from build123d import *

# Parameters (mm, degrees)
SKETCH1_R           = 1
BOSS_EXTRUDE1_DEPTH = 1
SKETCH2_R           = 1
BOSS_EXTRUDE2_DEPTH = 1
SKETCH3_R           = 1
BOSS_EXTRUDE3_DEPTH = 1


with BuildPart() as part:
    # Sketch1 → Boss-Extrude1 (new body)
    with BuildSketch(Plane(origin=(0, 0, 0), x_dir=(1, 0, 0), z_dir=(0, 1, 0))):
        with BuildLine():
            Line((-26.5, 3), (26.5, 3))
            ThreePointArc((26.5, 3), (29.222667474, 1.259794359), (28.786667416, -1.941945449))
            Line((28.786667416, -1.941945449), (2.247877744, -8.598102408))
            ThreePointArc((2.247877744, -8.598102408), (-0.45558898, -8.991146774), (-3.153897824, -8.56412735))
            Line((-3.153897824, -8.56412735), (-26.5, -3))
            ThreePointArc((-26.5, -3), (-29.5, 0), (-26.5, 3))
        make_face()
        with Locations((-26.5, 0)):
            Circle(SKETCH1_R, mode=Mode.SUBTRACT)
        with Locations((26.5, 0)):
            Circle(SKETCH1_R, mode=Mode.SUBTRACT)
        with Locations((-0.709607331, -6.824747005)):
            Circle(SKETCH1_R, mode=Mode.SUBTRACT)
    extrude(amount=BOSS_EXTRUDE1_DEPTH)



with BuildPart() as body_2:
    # Sketch2 → Boss-Extrude2 (new body)
    with BuildSketch(Plane(origin=(0, 1, 0), x_dir=(1, 0, 0), z_dir=(0, 1, 0))):
        with Locations((-26.5, 0)):
            Circle(SKETCH2_R)
    extrude(amount=BOSS_EXTRUDE2_DEPTH)


with BuildPart() as part_1:
    add(part.part)

    add(body_2.part)  # Boss-Extrude3 merges body 2
    # Sketch3 → Boss-Extrude3 (add)
    with BuildSketch(Plane.XZ):
        with Locations((-26.5, 0)):
            Circle(SKETCH3_R)
    extrude(amount=-BOSS_EXTRUDE3_DEPTH)


solid = part_1.part
Here's how the part is built. I have some questions about the finished solid (model axes, mm). A direction names the side the tool comes from. Round coordinates to 2 decimals unless told otherwise and drop trailing zeros. Loops run counter-clockwise (first coordinate to the right, second up) from the corner with the lowest first, then second, coordinate; pieces in that order, holes last.
1. For P1, Ø4, axis at x = -5, z = 1.5, coming from the +Y side, with a flat end and sliding along its axis, tell me the tip position at first contact or that it passes through.
Answer list:
P1: stops at y = 1
2. If we section it at C-C on x = -5: Write out the boundary of the cut face in (y, z), plus the area to 3 significant figures.
Answer list:
outline: (0, -3) - (1, -3) - (1, 8.12) - (0, 8.12) - close
area: 11.1 mm2
3. If I drill on line 1 along X through (y, z) = (0.7, 0); line 2 along Y through (x, z) = (23, 1.25); line 3 along Z through (x, y) = (26.5, 0.3), over which ranges is the centre line in solid material (lowest first)?
Answer list:
line 1: x = -29.5 to 25.5, 27.5 to 29.5
line 2: y = 0 to 1
line 3: z = -3 to -1, 1 to 2.52
4. If we section it at A-A on z = 0: Write out the boundary of the cut face in (x, y).
Answer list:
outline: (-29.5, 0) - (25.5, 0) - (25.5, 1) - (-25.5, 1) - (-25.5, 2) - (-27.5, 2) - (-27.5, 1) - (-29.5, 1) - close; (27.5, 0) - (29.5, 0) - (29.5, 1) - (27.5, 1) - close
5. If we section it at D-D on z = 5: Write out the boundary of the cut face in (x, y), plus the area to 3 significant figures.
Answer list:
outline: (-18.11, 0) - (16.59, 0) - (16.59, 1) - (-18.11, 1) - close
area: 34.7 mm2
6. We'd pull the mould along X, two halves only. Please class faces 3 (the face through (-0.248, 0.493, 7.712)), 4 (the face through (-27, 2, 0)), 5 (the face through (-14.66, 0.49, 5.82)), 6 (the face through (25.5, 0.5, 0)): +X half, -X half, draft (parallel to the pull), parting line (faces both ways), or undercut.
Answer list:
face 3: undercut
face 4: draft
face 5: -X half
face 6: undercut
7. If we section it at B-B on y = 0.5: Write out the boundary of the cut face in (x, z), plus the area to 3 significant figures.
Answer list:
outline: (-26.5, -3) - (26.5, -3) arc R3 ccw to (28.79, 1.94) - (2.25, 8.6) arc R9.1 ccw to (-3.15, 8.56) - (-26.5, 3) arc R3 ccw to start; hole circle Ø2 at (-0.71, 6.82); hole circle Ø2 at (26.5, 0)
area: 498 mm2
8. Which directions (+Z, -Z, +X, -X, +Y, -Y) give clear straight access to the entire face, cutting with the end or side of a thin tool? Please do faces 1 (the face through (-0.42, 0.49, 8.99)), 2 (the face through (-27.5, 1.5, 0)).
Answer list:
face 1: +Z, +Y, -Y
face 2: +Y
